Answer from the drawing. Dimensions are ordinates in mm from the lowest x, y and z of the part. Round coordinates to 2 decimals unless told otherwise and drop trailing zeros. Write each loop counter-clockwise with the first axis right and the second up, starting at its lowest first coordinate (ties: lowest second). Pieces come first, ordered by that corner, then holes. Notation, with made-up numbers: (28, 67.25) - (58, 67.25) arc R22 ccw to (58, 92.25) - close; hole circle Ø6 at (55.5, 24). An arc over 180 degrees is marked (long way). Write item = value, one per line. Start each with the question number.
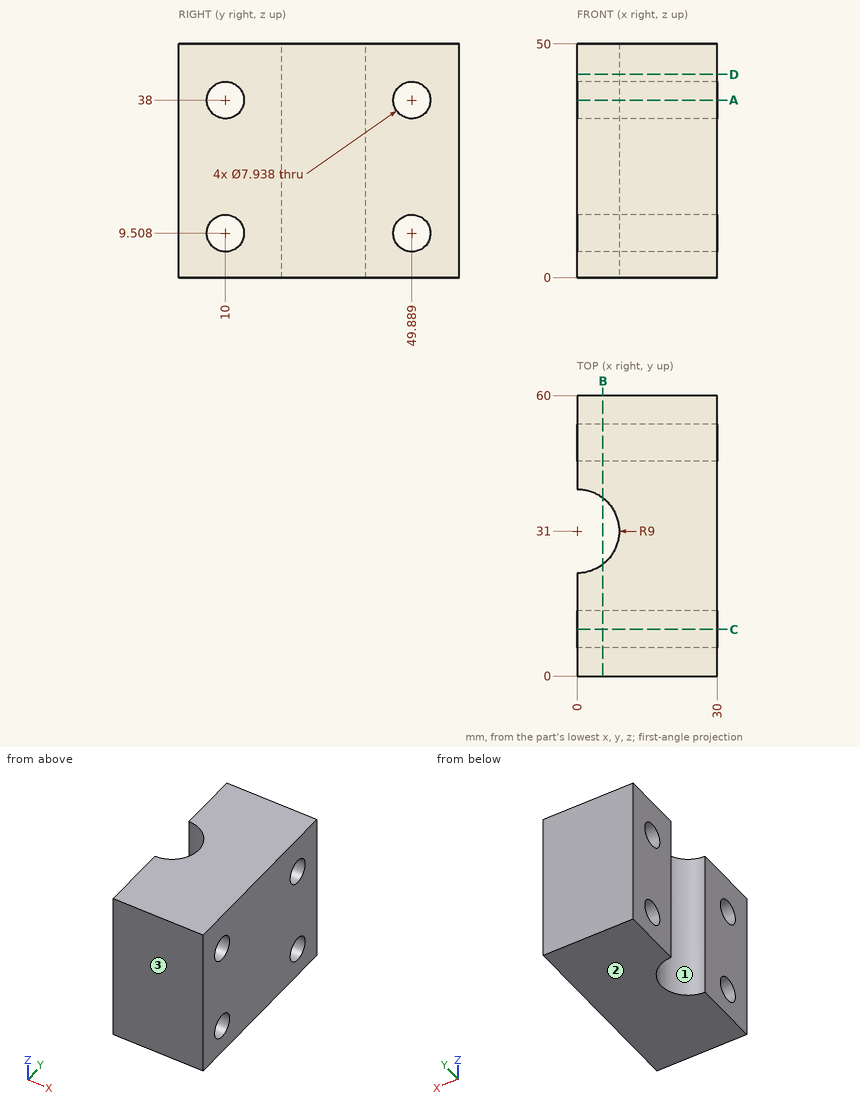
1. Find section B-B on x = 5.5. Give the vertices of the cut face in (y, z), plus the area to 3 significant figures.
2. Find section D-D on z = 43.5. Give the vertices of the cut face in (x, y), plus the area to 3 significant figures.
3. Consider line 1 (Z direction, x = 19, y = 10); line 2 (Y direction, x = 8.25, z = 41.5) (1 decimal); line 3 (Z direction, x = 25.5, y = 48). Determine where each line is inside the solid, lowest interval first.
4. Find section C-C on y = 10. Give the vertices of the cut face in (x, z).
5. For a pull along Y with two mould halves and no side action, classify the marked faces 1, 2 and 3 as released by +Y, released by -Y, zero draft, split by the parting line, or undercut.
6. Find section A-A on z = 38. Give the vertices of the cut face in (x, y).
Answer key:
q1.outline = (0, 0) - (23.88, 0) - (23.88, 50) - (0, 50) - close; (38.12, 0) - (60, 0) - (60, 50) - (38.12, 50) - close; hole circle Ø7.94 at (10, 9.51); hole circle Ø7.94 at (10, 38); hole circle Ø7.94 at (49.89, 9.51); hole circle Ø7.94 at (49.89, 38)
q1.area = 2,090 mm²
q2.outline = (0, 0) - (30, 0) - (30, 60) - (0, 60) - (0, 40) arc R9 cw to (0, 22) - close
q2.area = 1,670 mm²
q3.line_1 = 0 to 5.54, 13.48 to 34.03, 41.97 to 50
q3.line_2 = 0 to 8.1, 11.9 to 27.4, 34.6 to 48, 51.8 to 60
q3.line_3 = 0 to 6.02, 13 to 34.51, 41.49 to 50
q4.outline = (0, 0) - (30, 0) - (30, 5.54) - (0, 5.54) - close; (0, 13.48) - (30, 13.48) - (30, 34.03) - (0, 34.03) - close; (0, 41.97) - (30, 41.97) - (30, 50) - (0, 50) - close
q5.face_1 = undercut
q5.face_2 = zero draft
q5.face_3 = released by -Y
q6.outline = (0, 0) - (30, 0) - (30, 6.03) - (0, 6.03) - close; (0, 13.97) - (30, 13.97) - (30, 45.92) - (0, 45.92) - (0, 40) arc R9 cw to (0, 22) - close; (0, 53.86) - (30, 53.86) - (30, 60) - (0, 60) - close
